Work out the finished part from the listing and answer in its coordinate system (mm). A direction names the side the tool comes from. Round coordinates to 2 decimals unless told otherwise and drop trailing zeros. Use a Markdown table: item, result. Add a question column.
Item 1: For a pull along X with two mould halves and no side action, classify faces 3 (the flat face through (-11.446, -16, 12)), 4 (the cylindrical face through (-8.92, -33.365, 19.77)), 5 (the flat face through (81.554, -15, 12)) as +X half, -X half, draft (parallel to the pull), parting line (faces both ways), or undercut.
Item 2: Find the intervals of material crossed by L1, parallel to Y at x = -7, z = 20.75; L2, parallel to Y at x = -6, z = 21, in increasing order. Write a range as [from, to].
Item 3: A tool of negligible diameter and unlimited length cuts with its end or side. For faces 1 (the cylindrical face through (-9.444, 4.272, 19.77)), 2 (the flat face through (34, 8.184, 12)), from which of +Z, -Z, +X, -X, +Y, -Y can it reach the whole face along a straight path? Write none if from no direction.
Item 4: Flat-ended cylindrical pins translate along their axes: P1, Ø1.2, axis at x = -6.5, y = 4, coming from the +Z side; P2, Ø2.5, axis at x = -7.45, y = -15.27, coming from the -Z side. Find the tip coordinate at first contact, or state that the pin passes through.
Autodesk Inventor part; units mm, degrees
ref_plane "YZ Plane" through (0, 0, 0) normal (1, 0, 0) x (0, 1, 0)
ref_plane "XZ Plane" through (0, 0, 0) normal (0, 1, 0) x (-1, 0, 0)
ref_plane "XY Plane" through (0, 0, 0) normal (0, 0, 1) x (1, 0, 0)
sketch "スケッチ1" plane through (0, 0, 0) normal (0, 0, 1) x (1, 0, 0)
  line L0 (-11.4461, 8.1838) -> (81.5539, 8.1838)
  line L1 (81.5539, 8.1838) -> (81.5539, -38.7162)
  line L2 (81.5539, -38.7162) -> (-11.4461, -38.7162)
  line L3 (-11.4461, -38.7162) -> (-11.4461, 8.1838)
  point P0 (0, 0)
  dimension "d0" = 93
  dimension "d1" = 46.9
extrude "押し出し1" add sketch "スケッチ1" along normal blind 24.7
fillet "フィレット1" radius 1 12 edges at (35.0539, 8.1838, 24.7) (-11.4461, -15.2662, 24.7) (-11.4461, 8.1838, 12.35) (35.0539, -38.7162, 24.7) (-11.4461, -38.7162, 12.35) (35.0539, -38.7162, 0) (81.5539, -38.7162, 12.35) (81.5539, -15.2662, 24.7) (81.5539, 8.1838, 12.35) (81.5539, -15.2662, 0) (35.0539, 8.1838, 0) (-11.4461, -15.2662, 0)
sketch "スケッチ2" plane through (0, 0, 24.7) normal (0, 0, 1) x (1, 0, 0)
  line L0 (-10.4461, -37.7162) -> (-10.4461, 7.1838)
  line L1 (80.5539, -37.7162) -> (-10.4461, -37.7162)
  line L2 (80.5539, 7.1838) -> (80.5539, -37.7162)
  line L3 (-10.4461, 7.1838) -> (80.5539, 7.1838)
  circle A0 centre (-7.4461, 4.1838) radius 2
  circle A1 centre (-7.4461, -34.7162) radius 2
  line L4 (-0.4461, 2.1838) -> (75.5539, 2.1838)
  line L5 (75.5539, 2.1838) -> (75.5539, -32.7162)
  line L6 (75.5539, -32.7162) -> (-0.4461, -32.7162)
  line L7 (-0.4461, -32.7162) -> (-0.4461, 2.1838)
  circle A2 centre (-7.4461, -15.2662) radius 1
  point P0 (0, 0)
  dimension "d5" = 4
  dimension "d6" = 4
  dimension "d7" = 3
  dimension "d8" = 3
  dimension "d9" = 3
  dimension "d10" = 3
  dimension "d11" = 5
  dimension "d12" = 5
  dimension "d13" = 5
  dimension "d14" = 10
  dimension "d15" = 2
extrude "押し出し2" cut sketch "スケッチ2" against normal blind 10 contours A0 | A1 | A2
sketch "スケッチ3" plane through (0, 0, 24.7) normal (0, 0, 1) x (1, 0, 0)
  line L0 (-2.3175, 1.7393) -> (76.8469, 1.7393) construction
  line L1 (76.8469, 1.7393) -> (76.8469, -32.2836) construction
  line L2 (76.8469, -32.2836) -> (-2.3175, -32.2836) construction
  line L3 (-2.3175, -32.2836) -> (-2.3175, 1.7393) construction
  point P0 (0, 0)
properties part number "BAKUSO"
Reported:
| question | item | result |
|---|---|---|
| 1 | face 3 | -X half |
| 1 | face 4 | undercut |
| 1 | face 5 | +X half |
| 2 | L1 | [-38.72, -36.67], [-32.77, -16.16], [-14.37, 2.23], [6.13, 8.18] |
| 2 | L2 | [-38.72, -36.1], [-33.33, 2.8], [5.57, 8.18] |
| 3 | face 1 | +Z |
| 3 | face 2 | +Z, -Z, +X, -X, +Y |
| 4 | P1 | z = 14.7 |
| 4 | P2 | z = 0 |
